Check sheet for the modelled part. Datum: model origin and axes. Units: mm. A direction names the side the tool comes from. Coordinates: 2 decimals unless noted, no trailing zeros. Order: outer loops, then holes, each group sorted by start corner. A loop starts at its lowest first (then second) coordinate and runs counter-clockwise, first axis right, second up.
1. Cross-section at B-B (x = -18). Enter the section's corners in (y, z), then the cut area to 3 significant figures.
2. Cross-section at C-C (y = -66). Enter the section's corners in (x, z).
3. Gauge pin test, flat ends, axial feed: pin 1 Ø2.5 at (y, z) = (-65, 66.5) entering from -X; pin 2 Ø2 at (x, y) = (-22, -62.5) entering from -Z; pin 3 Ø3 at (x, z) = (28, 61.5) entering from -Y; pin 4 Ø1 at (y, z) = (-62, 155.5) entering from -X. Record the tip position at first contact, or that the pin passes through.
4. Thickness scan on line 1 (X direction, y = -65.25, z = 18); line 2 (Y direction, x = 5, z = 94.5); line 3 (Y direction, x = -33.5, z = 115). Record the ranges inside material, lowest first.
5. Set-up check for faces 1 (the flat face through (-1, -60, 0)), 2 (the flat face through (-2.54, -66, 85)), 3 (the flat face through (17, -63.64, 88)): record each of +Z, -Z, +X, -X, +Y, -Y from which the full face is reachable in a straight line by a thin tool's end or side.
6. Cross-section at A-A (z = 65). Enter the section's corners in (x, y).
```python
from build123d import *

# Parameters (mm, degrees)
SKETCH3_R           = 71.12
BOSS_EXTRUDE2_DEPTH = 172.72
CUT_EXTRUDE3_DEPTH  = 173.72
CUT_EXTRUDE4_DEPTH  = 173.72
SKETCH7_W           = 132.752189526
SKETCH7_H           = 172.72
CUT_EXTRUDE5_DEPTH  = 31.75
SKETCH8_W           = 5.08
SKETCH8_H           = 172.72
BOSS_EXTRUDE3_DEPTH = 5.08


with BuildPart() as part:
    # Sketch3 → Boss-Extrude2 (new body)
    with BuildSketch(Plane.XY):
        Circle(SKETCH3_R)
    extrude(amount=BOSS_EXTRUDE2_DEPTH)

    # Sketch4 → Cut-Extrude3 (cut, through all)
    with BuildSketch(Plane.XY.offset(172.72)):
        with BuildLine():
            Line((-31.75, -63.639546667), (31.75, -63.639546667))
            ThreePointArc((31.75, -63.639546667), (0, -71.12), (-31.75, -63.639546667))
        make_face()
    extrude(amount=-CUT_EXTRUDE3_DEPTH, mode=Mode.SUBTRACT)

    # Sketch5 → Cut-Extrude4 (cut, through all)
    with BuildSketch(Plane.XY.offset(172.72)):
        with BuildLine():
            Line((-66.376094763, -25.539546667), (66.376094763, -25.539546667))
            ThreePointArc((66.376094763, -25.539546667), (0, 71.12), (-66.376094763, -25.539546667))
        make_face()
    extrude(amount=-CUT_EXTRUDE4_DEPTH, mode=Mode.SUBTRACT)

    # Sketch7 → Cut-Extrude5 (cut)
    with BuildSketch(Plane(origin=(0, -25.539546667, 0), x_dir=(1, 0, 0), z_dir=(0, 1, 0))):
        with Locations((0, -86.36)):
            Rectangle(SKETCH7_W, SKETCH7_H)
    extrude(amount=-CUT_EXTRUDE5_DEPTH, mode=Mode.SUBTRACT)

    # Sketch8 → Boss-Extrude3 (add)
    with BuildSketch(Plane.XZ.offset(63.639546667)):
        with Locations((0, 86.36)):
            Rectangle(SKETCH8_W, SKETCH8_H)
    extrude(amount=BOSS_EXTRUDE3_DEPTH)


solid = part.part
```
Data:
1. outline: (-63.64, 0) - (-57.29, 0) - (-57.29, 172.72) - (-63.64, 172.72) - close
1. area: 1,100 mm2
2. outline: (-2.54, 0) - (2.54, 0) - (2.54, 172.72) - (-2.54, 172.72) - close
3. pin 1: stops at x = -2.54
3. pin 2: stops at z = 0
3. pin 3: stops at y = -63.64
3. pin 4: stops at x = -35.72
4. line 1: x = -2.54 to 2.54
4. line 2: y = -63.64 to -57.29
4. line 3: y = -62.74 to -57.29
5. face 1: -Z, +X, -X, +Y, -Y
5. face 2: +Z, -Z, -X, -Y
5. face 3: +Z, -Z, +X, -Y
6. outline: (-42.14, -57.29) arc R71.12 ccw to (-31.75, -63.64) - (-2.54, -63.64) - (-2.54, -68.72) - (2.54, -68.72) - (2.54, -63.64) - (31.75, -63.64) arc R71.12 ccw to (42.14, -57.29) - close
